Geometry: final body of the model. Coordinates: model frame, mm. A direction names the side the tool comes from. Give positions to 0.01 mm unless a question says otherwise; leave off trailing zeros. Loops run counter-clockwise (first coordinate to the right, second up) from the corner with the lowest first, then second, coordinate; pieces in that order, holes last. Notation, with made-up numbers: (7.5, 27.25) -> (27.5, 27.25) arc R14 cw to (27.5, 53.25) -> close; hole circle Ø7 at (-13, -36.5). An arc over 180 degrees is marked (long way). Answer in a Markdown table with one row per item. Add a question column.
Autodesk Inventor part; units mm, degrees
ref_plane "YZ Plane" through (0, 0, 0) normal (1, 0, 0) x (0, 1, 0)
ref_plane "XZ Plane" through (0, 0, 0) normal (0, 1, 0) x (-1, 0, 0)
ref_plane "XY Plane" through (0, 0, 0) normal (0, 0, 1) x (1, 0, 0)
sketch "Sketch2" plane through (0, 0, 0) normal (0, 0, 1) x (1, 0, 0)
  line L0 (39.8575, 12.7612) -> (31.599, 12.7612)
  line L1 (39.8575, 12.7612) -> (20.8075, 12.7612)
  line L2 (79.512, -31.9773) -> (79.512, 12.7612)
  line L3 (79.512, 12.7612) -> (37.4294, 12.7612)
  circle A0 centre (60.3451, -12.7) radius 2.54
  circle A1 centre (73.0451, -12.7) radius 2.54
  circle A2 centre (73.0451, -25.4) radius 2.54
  line L4 (92.334, -18.8499) -> (92.334, 1.5256)
  circle A3 centre (85.7451, -25.4) radius 3.9624
  circle A4 centre (85.7451, -12.7) radius 2.1844
  line L5 (25.7365, 2.0147) -> (43.2474, -39.355)
  line L6 (47.6451, -34.29) -> (41.1035, -34.29)
  line L7 (92.334, -18.8499) -> (92.334, -34.29)
  line L8 (47.6451, -34.29) -> (92.334, -34.29)
  line L9 (-341.1851, -3.2325) -> (91.1147, -3.2325)
  line L10 (25.7365, 2.0147) -> (20.8075, 12.7612)
  line L11 (91.1147, -3.2325) -> (92.334, -3.2325)
  circle A5 centre (85.7451, -25.4) radius 5.08
  point P0 (0, 0)
  point P1 (41.3274, -31.9773)
  point P2 (79.512, -18.8499)
  point P3 (79.512, -3.2325)
  dimension "d38" = 19.05
  dimension "d39" = 432.2999
  dimension "d40" = 10.16
extrude "Extrusion3" add sketch "Sketch2" along normal blind 1.5875 contours L3 L2 L9 L5 L10 L1 L0 | L9 L11 L4 L7 L8 L6 L5
fillet "Fillet9" radius 6.35 5 edges at (79.512, 12.7612, 0.7937) (79.512, -3.2325, 0.7937) (92.334, -3.2325, 0.7937) (92.334, -34.29, 0.7937) (41.1035, -34.29, 0.7937)
fillet "Fillet10" radius 1.5875 1 edges at (20.8075, 12.7612, 0.7937)
properties part number "Sleds poly V3"
(1) Material intervals for line 1 along Y through (x, z) = (71.5, 0.7); line 2 along X through (y, z) = (-13.5, 0.6); line 3 along Y through (x, z) = (74, 0.85), sorted ascending. Write a range as from..to.
(2) Cut plane D-D on x = 40.5. Return the cut outline in (y, z), then the cut area to 3 significant figures.
(3) Reachability of faces 4 (the cylindrical face through (75.47, -13.46, 0.78)), 5 (the flat face through (79.512, 5, 1)) from +Z, -Z, +X, -X, +Y, -Y: full face, straight path, thin tool, end or side. Return the list, or none.
(4) Draft query along Y for faces 1 (the cylindrical face through (21.96, 12.05, 0.8)), 2 (the cylindrical face through (41.76, -33.204, 0.805)), 3 (the cylindrical face through (80.67, -25.62, 0.78)). Return one class per face: +Y half, -Y half, draft (parallel to the pull), parting line (faces both ways), or undercut.
(5) Cut plane A-A on y = -25.4. Return the cut outline in (x, z), then the cut area to 3 significant figures.
(6) Cut plane B-B on z = 0.45. State how many separate pieces and enclosed holes the cut face has, then the cut area to 3 significant figures.
(7) Cut plane C-C on y = -12.7. Return the cut outline in (x, z), then the cut area to 3 significant figures.
Answer list:
| question | item | result |
|---|---|---|
| 1 | line 1 | y = -34.29..-27.42, -23.38..-14.72, -10.68..12.76 |
| 1 | line 2 | x = 32.3..57.93, 62.76..70.63, 75.46..83.71, 87.78..92.33 |
| 1 | line 3 | y = -34.29..-27.75, -23.05..-15.05, -10.35..12.71 |
| 2 | outline | (-32.08, 0) -> (12.76, 0) -> (12.76, 1.59) -> (-32.08, 1.59) -> close |
| 2 | area | 71.2 mm² |
| 3 | face 4 | +Z, -Z |
| 3 | face 5 | +Z, -Z, +X, +Y |
| 4 | face 1 | parting line |
| 4 | face 2 | -Y half |
| 4 | face 3 | undercut |
| 5 | outline | (37.34, 0) -> (70.51, 0) -> (70.51, 1.59) -> (37.34, 1.59) -> close; (75.59, 0) -> (80.67, 0) -> (80.67, 1.59) -> (75.59, 1.59) -> close; (90.83, 0) -> (92.33, 0) -> (92.33, 1.59) -> (90.83, 1.59) -> close |
| 5 | area | 63.1 mm² |
| 6 | separate pieces | 1 |
| 6 | enclosed holes | 5 |
| 6 | area | 2,500 mm² |
| 7 | outline | (31.96, 0) -> (57.81, 0) -> (57.81, 1.59) -> (31.96, 1.59) -> close; (62.89, 0) -> (70.51, 0) -> (70.51, 1.59) -> (62.89, 1.59) -> close; (75.59, 0) -> (83.56, 0) -> (83.56, 1.59) -> (75.59, 1.59) -> close; (87.93, 0) -> (92.33, 0) -> (92.33, 1.59) -> (87.93, 1.59) -> close |
| 7 | area | 72.8 mm² |
